Read the model definition and answer for the solid it produces. Units are mm, in the model's axes. A direction names the side the tool comes from. Round coordinates to 2 decimals unless told otherwise and drop trailing zeros. Order: outer loops, then holes, each group sorted by start corner. A loop starts at its lowest first (then second) coordinate and runs counter-clockwise, first axis right, second up. Notation, with made-up numbers: (-10, -4.75) - (29, -4.75) arc R12 cw to (29, 16.25) - close; hole circle Ø11 at (49.5, 79). An arc over 180 degrees is marked (long way). One line per question, with ' | ' between items. Start each with the question number.
1) For faces 4 (the cylindrical face through (9.015, 10.692, 1.706)), 5 (the flat face through (1, 2.2, 1)), determine the directions among +Z, -Z, +X, -X, +Y, -Y from which every point of the face is accessible in a straight line to the end or side of a thin tool.
2) The part is cut by section B-B, the plane x = -7.1. Give the vertices of the cut face in (y, z), plus the area to 3 significant figures.
3) The part is cut by section C-C, the plane y = 12. Give the vertices of the cut face in (x, z), plus the area to 3 significant figures.
4) Straight lines are drawn through the part: line 1 (Y direction, x = 8.9, z = 0); line 2 (X direction, y = 1.3, z = 0); line 3 (Z direction, x = -7.1, y = 0.75). For each, find the intervals that lie inside material, in ascending order. Write a range as from..to.
5) The mould has two halves that part along Y. Classify faces 1 (the flat face through (9, 18, 0)), 2 (the flat face through (7.9, 10, 1.5)), 3 (the cylindrical face through (9.02, 8.13, 0.28)): pulls with the +Y half, pulls with the -Y half, needs draft (parallel to the pull), parting line crosses it, or undercut.
6) A flat-ended cylindrical pin translates along its axis: pin 1 (2 mm diameter, centred on y = 16, z = 0, fed in from -X). Find the tip coordinate at first contact, or state that the pin passes through.
7) The part is cut by section A-A, the plane z = 0. Give the vertices of the cut face in (x, y).
8) The part is cut by section D-D, the plane z = 1.75. Give the vertices of the cut face in (x, y).
Autodesk Inventor part; units mm, degrees
ref_plane "YZ Plane" through (0, 0, 0) normal (1, 0, 0) x (0, 1, 0)
ref_plane "XZ Plane" through (0, 0, 0) normal (0, 1, 0) x (-1, 0, 0)
ref_plane "XY Plane" through (0, 0, 0) normal (0, 0, 1) x (1, 0, 0)
sketch "Sketch1" plane through (0, 0, 0) normal (0, 1, 0) x (-1, 0, 0)
  line L0 (-10.1, 3.25) -> (10.1, 3.25)
  line L1 (10.1, 3.25) -> (10.1, -3.25)
  line L2 (10.1, -3.25) -> (-10.1, -3.25)
  line L3 (-10.1, -3.25) -> (-10.1, 3.25)
  line L4 (0, 0) -> (0, -7.2216) construction
  line L5 (0, 0) -> (18.1335, 0) construction
  dimension "d0" = 6.5
  dimension "d1" = 20.2
extrude "Extrusion1" add sketch "Sketch1" along normal blind 2.2
sketch "Sketch2" plane through (0, 2.2, 0) normal (0, 1, 0) x (1, 0, 0)
  line L0 (-10.1, -3.25) -> (10.1, -3.25)
  line L1 (10.1, -3.25) -> (10.1, 3.25)
  line L2 (10.1, 3.25) -> (-10.1, 3.25)
  line L3 (-10.1, 3.25) -> (-10.1, -3.25)
  line L4 (7.9, 3.25) -> (7.9, -3.25) construction
  line L5 (-1.1, 6.7296) -> (-1.1, -8.5112) construction
  circle A0 centre (-1.1, 0) radius 2.15
  circle A1 centre (-7.1, 0) radius 2.15
  circle A2 centre (4.9, 0) radius 2.15
  circle A3 centre (-1.1, 0) radius 2.15
  point P0 (0, 0)
  dimension "d4" = 2.2
  dimension "d5" = 4.3
  dimension "d8" = 6
  dimension "d11" = 6
extrude "Extrusion2" cut sketch "Sketch2" against normal through all contours A0 | A1 | A2
sketch "Sketch3" plane through (0, 2.2, 0) normal (0, 1, 0) x (1, 0, 0)
  line L0 (10.1, 3.25) -> (-10.1, 3.25)
  line L1 (7.9, 3.25) -> (10.1, 3.25)
  line L2 (10.1, 3.25) -> (10.1, -3.25)
  line L3 (10.1, -3.25) -> (7.9, -3.25)
  line L4 (7.9, -3.25) -> (7.9, 3.25)
  point P0 (0, 0)
  dimension "d19" = 2.2
extrude "Extrusion3" add sketch "Sketch3" along normal blind 15.8
sketch "Sketch4" plane through (10.1, 0, 3.25) normal (1, 0, 0) x (0, 0, -1)
  line L0 (0, 0) -> (0, 18)
  line L1 (3.25, 19.7577) -> (3.25, -0.3358) construction
  circle A0 centre (3.25, 6) radius 2.15
  circle A1 centre (3.25, 12) radius 2.15
  point P0 (3.25, 0)
  dimension "d22" = 4.3
  dimension "d23" = 4.3
  dimension "d24" = 6
  dimension "d25" = 6
extrude "Extrusion4" cut sketch "Sketch4" against normal through all
equation "\"d2\" = Depth"
equation "\"d4\" = Depth"
equation "\"d5\" = Holes"
equation "\"d17\" = Depth"
equation "\"d19\" = Depth"
equation "\"d22\" = Holes"
equation "\"d23\" = Holes"
equation "\"Holes\" = 4.3"
equation "\"Depth\" = 2.2"
properties part number "Equerre"
Values:
1) face 4: +X, -X | face 5: +Z, -Z, -X, +Y
2) outline: (0, -3.25) - (2.2, -3.25) - (2.2, -2.15) - (0, -2.15) - close; (0, 2.15) - (2.2, 2.15) - (2.2, 3.25) - (0, 3.25) - close | area: 4.84 mm^2
3) outline: (7.9, -3.25) - (10.1, -3.25) - (10.1, -2.15) - (7.9, -2.15) - close; (7.9, 2.15) - (10.1, 2.15) - (10.1, 3.25) - (7.9, 3.25) - close | area: 4.84 mm^2
4) line 1: y = 0..3.85, 8.15..9.85, 14.15..18 | line 2: x = -10.1..-9.25, -4.95..-3.25, 1.05..2.75, 7.05..10.1 | line 3: z = -3.25..-2.15, 2.15..3.25
5) face 1: pulls with the +Y half | face 2: needs draft | face 3: undercut
6) pin 1: stops at x = 7.9
7) outline: (-10.1, 0) - (-9.25, 0) - (-9.25, 2.2) - (-10.1, 2.2) - close; (-4.95, 0) - (-3.25, 0) - (-3.25, 2.2) - (-4.95, 2.2) - close; (1.05, 0) - (2.75, 0) - (2.75, 2.2) - (1.05, 2.2) - close; (7.05, 0) - (10.1, 0) - (10.1, 3.85) - (7.9, 3.85) - (7.9, 2.2) - (7.05, 2.2) - close; (7.9, 8.15) - (10.1, 8.15) - (10.1, 9.85) - (7.9, 9.85) - close; (7.9, 14.15) - (10.1, 14.15) - (10.1, 18) - (7.9, 18) - close
8) outline: (-10.1, 0) - (-8.35, 0) - (-8.35, 2.2) - (-10.1, 2.2) - close; (-5.85, 0) - (-2.35, 0) - (-2.35, 2.2) - (-5.85, 2.2) - close; (0.15, 0) - (3.65, 0) - (3.65, 2.2) - (0.15, 2.2) - close; (6.15, 0) - (10.1, 0) - (10.1, 4.75) - (7.9, 4.75) - (7.9, 2.2) - (6.15, 2.2) - close; (7.9, 7.25) - (10.1, 7.25) - (10.1, 10.75) - (7.9, 10.75) - close; (7.9, 13.25) - (10.1, 13.25) - (10.1, 18) - (7.9, 18) - close
